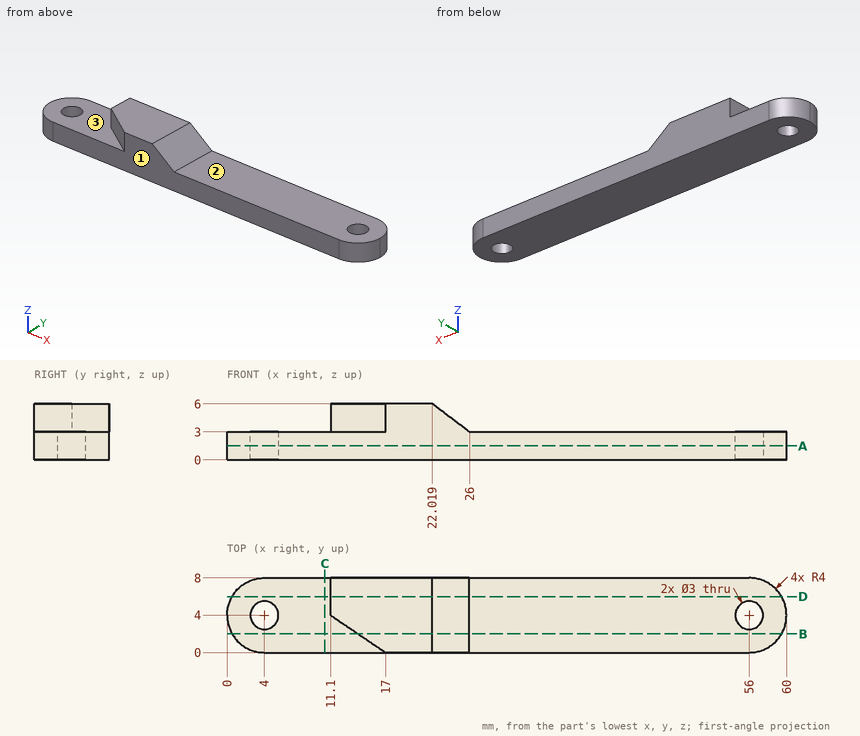
Geometry check sheet. Reference: drawing and pictorial views, mm from the part's lowest x, y, z. A direction names the side the tool comes from. Give positions to 0.01 mm unless a question says otherwise; leave off trailing zeros. Loops run counter-clockwise (first coordinate to the right, second up) from the corner with the lowest first, then second, coordinate; pieces in that order, holes last.
1. Section check C-C, the plane x = 10.5. Enter the section's corners in (y, z), then the cut area to 3 significant figures.
2. Go/stop test with flat-tipped pins: pin 1 Ø1.5 at (y, z) = (5.5, 4.5) entering from +X (1 decimal); pin 2 Ø3.5 at (x, y) = (4, 4) entering from +Z; pin 3 Ø0.9 at (y, z) = (7, 4.5) entering from -X. Record where each tip stops, or that it passes through.
3. Section check B-B, the plane y = 2. Enter the section's corners in (x, z).
4. Section check D-D, the plane y = 6. Enter the section's corners in (x, z), then the cut area to 4 significant figures.
5. Section check A-A, the plane z = 1.5. Count the separate pieces of the cut face and the enclosed holes in it, then the cut area to 3 significant figures.
6. Thickness scan on line 1 (Y direction, x = 56, z = 1.95); line 2 (X direction, y = 4.5, z = 2.5); line 3 (Z direction, x = 9, y = 2). Record the ranges inside material, lowest first.
7. Set-up check for the marked faces 1, 2 and 3: record each of +Z, -Z, +X, -X, +Y, -Y from which the full face is reachable in a straight line by a thin tool's end or side.
Geometry says:
1. outline: (0, 0) - (8, 0) - (8, 3) - (0, 3) - close
1. area: 24.0 mm2
2. pin 1: stops at x = 25
2. pin 2: stops at z = 3
2. pin 3: stops at x = 11.1
3. outline: (0.54, 0) - (59.46, 0) - (59.46, 3) - (26, 3) - (22.02, 6) - (14.05, 6) - (14.05, 3) - (0.54, 3) - close
4. outline: (0.54, 0) - (59.46, 0) - (59.46, 3) - (26, 3) - (22.02, 6) - (11.1, 6) - (11.1, 3) - (0.54, 3) - close
4. area: 215.5 mm2
5. separate pieces: 1
5. enclosed holes: 2
5. area: 452 mm2
6. line 1: y = 0 to 2.5, 5.5 to 8
6. line 2: x = 0.03 to 2.59, 5.41 to 54.59, 57.41 to 59.97
6. line 3: z = 0 to 3
7. face 1: +Z, -Z, +X, -X, -Y
7. face 2: +Z, +X, +Y, -Y
7. face 3: +Z, -X, -Y
